Could you check a few things on this model? Use its own coordinates, in mm. Give positions to 0.01 mm unless a question says otherwise; leave off trailing zeros. Order: outer loops, then holes, each group sorted by start corner. A loop starts at its lowest first (then second) coordinate and runs counter-clockwise, first axis right, second up.
from build123d import *

# Parameters (mm, degrees)
SKETCH1_R               = 2.0828
BOSS_EXTRUDE1_DEPTH     = 1.5875
SKETCH5_OUTSIDE_W       = 42.524
SKETCH5_OUTSIDE_H       = 43.874
SKETCH5_OUTSIDE_R       = 4.365625
CUT_EXTRUDE2_DEPTH      = 8.385856901
CUT_EXTRUDE2_DRAFT      = -60
MIRROR1_COPY_1_SKETCH_W = 42.524
MIRROR1_COPY_1_SKETCH_H = 43.874
MIRROR1_COPY_1_SKETCH_R = 4.365625
MIRROR1_COPY_1_DEPTH    = 8.385856901
MIRROR1_COPY_1_DRAFT    = -60


with BuildPart() as part:
    # Sketch1 → Boss-Extrude1 (new, symmetric)
    with BuildSketch(Plane(origin=(0, 0, 0), x_dir=(1, 0, 0), z_dir=(0, 1, 0))):
        Polygon((-4.365625, 2.520494769), (-4.365625, -2.520494769), (0, -5.040989538), (4.365625, -2.520494769), (4.365625, 2.520494769), (0, 5.040989538), align=None)
        with Locations(Location((0, 0, 0), (0, 0, 270))):
            Circle(SKETCH1_R, mode=Mode.SUBTRACT)
    extrude(amount=BOSS_EXTRUDE1_DEPTH, both=True)


with BuildPart() as cut_extrude2_tool:
    # Sketch5 outside → Cut-Extrude2 (with draft: the straight prism first)
    with BuildSketch(Plane(origin=(0, 1.5875, 0), x_dir=(1, 0, 0), z_dir=(0, 1, 0))):
        Rectangle(SKETCH5_OUTSIDE_W, SKETCH5_OUTSIDE_H)
        Circle(SKETCH5_OUTSIDE_R, mode=Mode.SUBTRACT)
    extrude(amount=-CUT_EXTRUDE2_DEPTH)
    # Cut-Extrude2: the draft: its side faces are tilted about the plane it starts from
    cut_extrude2_sides = [cut_extrude2_tool.faces().sort_by_distance(p)[0] for p in [
        (0, -2.60542845, 21.937),
        (21.262, -2.60542845, 0),
        (0, -2.60542845, -21.937),
        (-21.262, -2.60542845, 0),
        (-4.365625, -2.60542845, 0),
    ]]
    draft(cut_extrude2_sides, Plane(origin=(0, 1.5875, 0), x_dir=(1, 0, 0), z_dir=(0, 1, 0)), CUT_EXTRUDE2_DRAFT)


with BuildPart() as part_1:
    add(part.part)

    # Cut-Extrude2: cut by cut_extrude2_tool
    add(cut_extrude2_tool.part, mode=Mode.SUBTRACT)


with BuildPart() as mirror1_copy_1_tool:
    # Mirror1 copy 1 sketch → Mirror1 copy 1 (with draft: the straight prism first)
    with BuildSketch(Plane.XZ.offset(1.5875)):
        Rectangle(MIRROR1_COPY_1_SKETCH_W, MIRROR1_COPY_1_SKETCH_H)
        Circle(MIRROR1_COPY_1_SKETCH_R, mode=Mode.SUBTRACT)
    extrude(amount=-MIRROR1_COPY_1_DEPTH)
    # Mirror1 copy 1: the draft: its side faces are tilted about the plane it starts from
    mirror1_copy_1_sides = [mirror1_copy_1_tool.faces().sort_by_distance(p)[0] for p in [
        (0, 2.60542845, 21.937),
        (21.262, 2.60542845, 0),
        (0, 2.60542845, -21.937),
        (-21.262, 2.60542845, 0),
        (-4.365625, 2.60542845, 0),
    ]]
    draft(mirror1_copy_1_sides, Plane.XZ.offset(1.5875), MIRROR1_COPY_1_DRAFT)


with BuildPart() as part_2:
    add(part_1.part)

    # Mirror1 copy 1: cut by mirror1_copy_1_tool
    add(mirror1_copy_1_tool.part, mode=Mode.SUBTRACT)


solid = part_2.part
Item 1: Imagine slicing it at B-B on y = 1.4. List the corners of the cut face in (x, z) for me.
Findings:
outline: (-4.37, -1.71) arc R4.69 ccw to (-3.67, -2.92) - (-0.7, -4.64) arc R4.69 ccw to (0.7, -4.64) - (3.67, -2.92) arc R4.69 ccw to (4.37, -1.71) - (4.37, 1.71) arc R4.69 ccw to (3.67, 2.92) - (0.7, 4.64) arc R4.69 ccw to (-0.7, 4.64) - (-3.67, 2.92) arc R4.69 ccw to (-4.37, 1.71) - close; hole circle Ø4.17 at (0, 0)
Item 2: We'd pull the mould along X, two halves only. Please class faces 1 (the flat face through (2.213, 0.022, -3.763)), 2 (the flat face through (-4.366, 0, 0)), 3 (the cylindrical face through (0.626, -0.022, 1.987)): +X half, -X half, draft (parallel to the pull), parting line (faces both ways), or undercut.
Findings:
face 1: +X half
face 2: -X half
face 3: undercut
Item 3: For pin 1 (3.5 mm diameter, centred on x = 0, z = 0, fed in from -Y); pin 2 (1.5 mm diameter, centred on x = 1, y = 1, fed in from -Z), each with a flat end and sliding along its axis, tell me the tip position at first contact or that it passes through.
Findings:
pin 1: passes through
pin 2: stops at z = -4.9
Item 4: Please list where these lines run through material, in increasing order: line 1 along X through (y, z) = (-0.7, 0); line 2 along X through (y, z) = (0.55, -0.5); line 3 along Z through (x, y) = (-1, 0.55).
Findings:
line 1: x = -4.37 to -2.08, 2.08 to 4.37
line 2: x = -4.37 to -2.02, 2.02 to 4.37
line 3: z = -4.46 to -1.83, 1.83 to 4.46
Item 5: Imagine slicing it at A-A on y = -0.2. List the corners of the cut face in (x, z) for me.
Findings:
outline: (-4.37, -2.52) - (0, -5.04) - (4.37, -2.52) - (4.37, 2.52) - (0, 5.04) - (-4.37, 2.52) - close; hole circle Ø4.17 at (0, 0)
